Design review of the part shown in the three views and the two pictorial views. Dimensions are in mm from the part's minimum x, y and z. A direction names the side the tool comes from. Coordinates: 2 decimals unless noted, no trailing zeros. Write each loop counter-clockwise with the first axis right and the second up, starting at its lowest first coordinate (ties: lowest second). Pieces come first, ordered by that corner, then holes. Notation, with made-up numbers: (39.25, 48.25) -> (43.25, 48.25) arc R23 cw to (43.25, 64.25) -> close; hole circle Ø10 at (-4, 76.25). An arc over 180 degrees is marked (long way). Write each question's results on one line, items separated by ' | '.
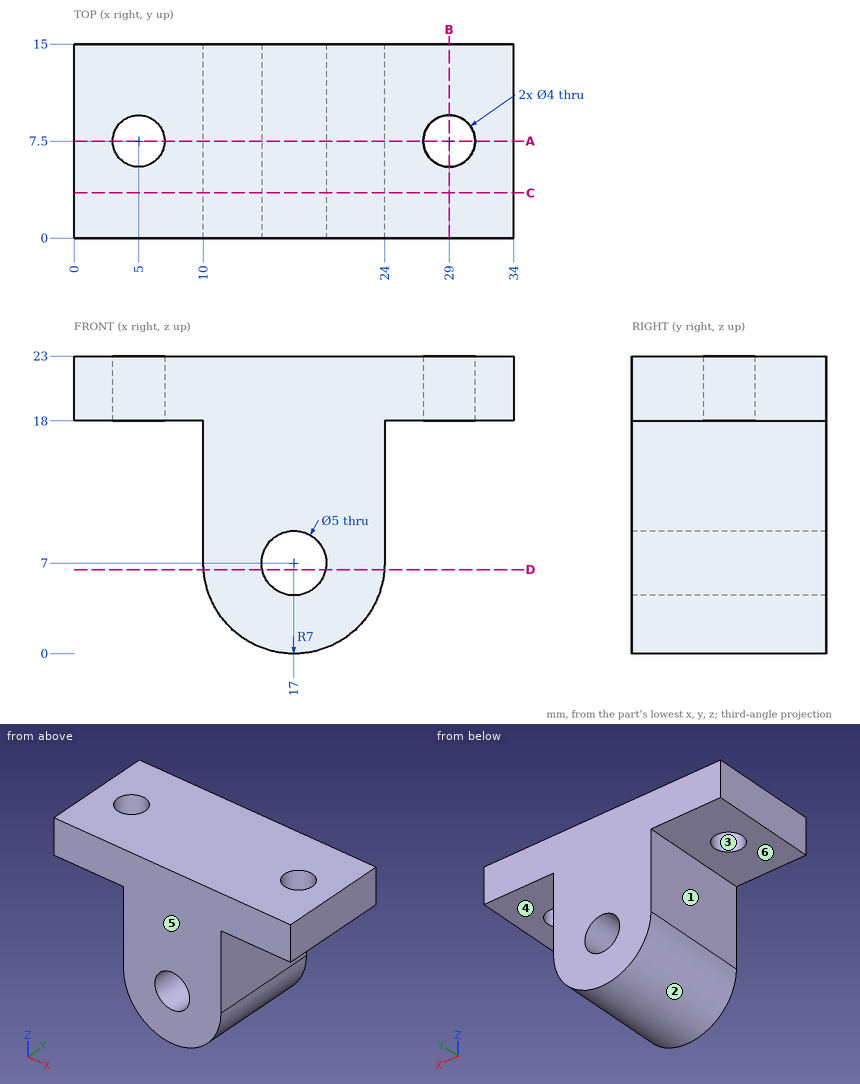
Q1. Add section D-D (z = 6.5). Write out the cut boundary in (x, y), plus the area to 3 significant figures.
Solution:
outline: (10.02, 0) -> (14.55, 0) -> (14.55, 15) -> (10.02, 15) -> close; (19.45, 0) -> (23.98, 0) -> (23.98, 15) -> (19.45, 15) -> close | area: 136 mm²
Q2. For line 1 (X direction, y = 8, z = 7); line 2 (Y direction, x = 5, z = 19.9); line 3 (Z direction, x = 2.5, y = 9), list the stretches that pass through material, from the lowest coordinate up. Write a range as from..to.
Solution:
line 1: 10..14.5, 19.5..24 | line 2: 0..5.5, 9.5..15 | line 3: 18..23
Q3. Machinability: for the marked faces 4, 5 and 6, which of the approach directions +Z, -Z, +X, -X, +Y, -Y give a long, thin tool a straight path to every point of the face, cutting with its end or side? Answer none if there is none.
Solution:
face 4: -Z, +X, +Y, -Y | face 5: +Z, -Z, +X, -X, -Y | face 6: -Z, -X, +Y, -Y
Q4. Add section C-C (y = 3.5). Write out the cut boundary in (x, z).
Solution:
outline: (0, 18) -> (10, 18) -> (10, 7) arc R7 ccw to (24, 7) -> (24, 18) -> (34, 18) -> (34, 23) -> (0, 23) -> close; hole circle Ø5 at (17, 7)
Q5. Clearance check with flat-ended pins moving along their axes: P1, Ø5.5, axis at y = 10, z = 12, coming from the -X side; P2, Ø5, axis at y = 5.5, z = 2.5, coming from the -X side; P3, Ø1, axis at x = 23, y = 6, coming from the -Z side; P4, Ø4, axis at y = 9.5, z = 17.5, coming from the -X side. State where each tip first meets the part, or that it passes through.
Solution:
P1: x = 10 | P2: x = 10.29 | P3: z = 2.67 | P4: x = 0
Q6. Add section B-B (x = 29). Write out the cut boundary in (y, z), plus the area to 3 significant figures.
Solution:
outline: (0, 18) -> (5.5, 18) -> (5.5, 23) -> (0, 23) -> close; (9.5, 18) -> (15, 18) -> (15, 23) -> (9.5, 23) -> close | area: 55.0 mm²
Q7. Draft analysis for pull direction X (two halves, no side actions). For the marked faces 1, 2 and 3, state which applies: pulls with the +X half, pulls with the -X half, needs draft (parallel to the pull), parting line crosses it, or undercut.
Solution:
face 1: pulls with the -X half | face 2: parting line crosses it | face 3: undercut
Q8. Add section A-A (y = 7.5). Write out the cut boundary in (x, z), plus the area to 3 significant figures.
Solution:
outline: (0, 18) -> (3, 18) -> (3, 23) -> (0, 23) -> close; (7, 18) -> (10, 18) -> (10, 7) arc R7 ccw to (24, 7) -> (24, 18) -> (27, 18) -> (27, 23) -> (7, 23) -> close; (31, 18) -> (34, 18) -> (34, 23) -> (31, 23) -> close; hole circle Ø5 at (17, 7) | area: 341 mm²
